Part model, mm, in its own coordinate system. Face numbers are marked on the shaded views. Round coordinates to 2 decimals unless told otherwise and drop trailing zeros. Write each loop counter-clockwise with the first axis right and the second up, starting at its lowest first coordinate (ties: lowest second). Pieces come first, ordered by that corner, then holes. Notation, with made-up numbers: M 2.25,65.5 L 56.25,65.5 A25 ccw 56.25,88.5 Z; hole C 7.5,56 d8. An arc over 180 degrees is marked long. Use one line per item in the form item = value. Start each with the question number.
Item 1: Probe L1, parallel to X at y = 4, z = -9.5; L2, parallel to Y at x = 26, z = 26; L3, parallel to Z at x = 29, y = 6. List the from-to ranges inside material, lowest first.
Item 2: Flat gauge pins, fed straight in: pin 1 Ø6 at (x, z) = (-36, 11) entering from +Y; pin 2 Ø8 at (x, z) = (4, -23.5) entering from +Y; pin 3 Ø3 at (x, y) = (20.5, 12) entering from +Z. Where does each tip first touch, or does it go through?
Item 3: Cut at A-A, the plane y = 40. Give the cut face in (x, z).
Item 4: Cut at B-B, the plane z = -63. Give the cut face in (x, y), then the cut area to 3 significant figures.
Item 5: Mould opens along X. For the marked faces 1, 2, 3 and 4 say: +X half, -X half, draft (parallel to the pull), parting line (faces both ways), or undercut.
from build123d import *

# Parameters (mm, degrees)
SKETCH1_W           = 84
SKETCH1_H           = 155
BOSS_EXTRUDE1_DEPTH = 3
SKETCH2_W           = 3
SKETCH2_H           = 3
CUT_EXTRUDE1_DEPTH  = 3
SKETCH3_W           = 5
SKETCH3_H           = 8
BOSS_EXTRUDE2_DEPTH = 155
SKETCH4_W           = 5
SKETCH4_H           = 8
BOSS_EXTRUDE3_DEPTH = 155
SKETCH5_W           = 5
SKETCH5_H           = 58
BOSS_EXTRUDE4_DEPTH = 84
BOSS_EXTRUDE5_DEPTH = 5
BOSS_EXTRUDE6_DEPTH = 5
SKETCH8_W           = 84
SKETCH8_H           = 8
BOSS_EXTRUDE8_DEPTH = 5
SKETCH10_W          = 10
SKETCH10_H          = 7.49718506
CUT_EXTRUDE2_DEPTH  = 5
SKETCH11_W          = 10
SKETCH11_H          = 10.666578164
CUT_EXTRUDE3_DEPTH  = 5
SKETCH12_W          = 2.991300293
SKETCH12_H          = 5
CUT_EXTRUDE4_DEPTH  = 1.5
CUT_EXTRUDE5_DEPTH  = 1.5


with BuildPart() as part:
    # Sketch1 → Boss-Extrude1 (new body)
    with BuildSketch(Plane(origin=(0, 0, 0), x_dir=(1, 0, 0), z_dir=(0, 1, 0))):
        Rectangle(SKETCH1_W, SKETCH1_H)
    extrude(amount=BOSS_EXTRUDE1_DEPTH)

    # Sketch2 → Cut-Extrude1 (cut)
    with BuildSketch(Plane(origin=(0, 3, 0), x_dir=(1, 0, 0), z_dir=(0, 1, 0))):
        with Locations((35.5, -71)):
            Rectangle(SKETCH2_W, SKETCH2_H)
        with Locations((-35.5, -71)):
            Rectangle(SKETCH2_W, SKETCH2_H)
    extrude(amount=-CUT_EXTRUDE1_DEPTH, mode=Mode.SUBTRACT)

    # Sketch3 → Boss-Extrude2 (add)
    with BuildSketch(Plane.XY.offset(77.5)):
        with Locations((39.5, 4)):
            Rectangle(SKETCH3_W, SKETCH3_H)
    extrude(amount=-BOSS_EXTRUDE2_DEPTH)

    # Sketch4 → Boss-Extrude3 (add)
    with BuildSketch(Plane.XY.offset(77.5)):
        with Locations((-39.5, 4)):
            Rectangle(SKETCH4_W, SKETCH4_H)
    extrude(amount=-BOSS_EXTRUDE3_DEPTH)

    # Sketch5 → Boss-Extrude4 (add)
    with BuildSketch(Plane.ZY.offset(42)):
        with Locations((-75, 29)):
            Rectangle(SKETCH5_W, SKETCH5_H)
    extrude(amount=-BOSS_EXTRUDE4_DEPTH)

    # Sketch6 → Boss-Extrude5 (add)
    with BuildSketch(Plane.ZY.offset(42)):
        Polygon((-72.5, 58), (-22.5, 8), (-74.300026141, 4.41684906), (-74.300026141, 56.199973859), align=None)
    extrude(amount=-BOSS_EXTRUDE5_DEPTH)

    # Sketch7 → Boss-Extrude6 (add)
    with BuildSketch(Plane(origin=(42, 0, 0), x_dir=(0, 0, -1), z_dir=(1, 0, 0))):
        Polygon((72.5, 58), (19.108860597, 4.608860597), (75.247556584, 4.608860597), (75.247556584, 53.916409465), align=None)
    extrude(amount=-BOSS_EXTRUDE6_DEPTH)

    # Sketch8 → Boss-Extrude8 (add)
    with BuildSketch(Plane.XY.offset(77.5)):
        with Locations((0, 4)):
            Rectangle(SKETCH8_W, SKETCH8_H)
    extrude(amount=-BOSS_EXTRUDE8_DEPTH)

    # Sketch10 → Cut-Extrude2 (cut)
    with BuildSketch(Plane.XY.offset(77.5)):
        with Locations((-17, 6.74859253)):
            Rectangle(SKETCH10_W, SKETCH10_H)
    extrude(amount=-CUT_EXTRUDE2_DEPTH, mode=Mode.SUBTRACT)

    # Sketch11 → Cut-Extrude3 (cut)
    with BuildSketch(Plane.XY.offset(77.5)):
        with Locations((17, 8.333289082)):
            Rectangle(SKETCH11_W, SKETCH11_H)
    extrude(amount=-CUT_EXTRUDE3_DEPTH, mode=Mode.SUBTRACT)

    # Sketch12 → Cut-Extrude4 (cut)
    with BuildSketch(Plane(origin=(0, 0, 0), x_dir=(-1, 0, 0), z_dir=(0, -1, 0))):
        with Locations((35.504349854, -75)):
            Rectangle(SKETCH12_W, SKETCH12_H)
    extrude(amount=-CUT_EXTRUDE4_DEPTH, mode=Mode.SUBTRACT)

    # Sketch13 → Cut-Extrude5 (cut)
    with BuildSketch(Plane(origin=(0, 0, 0), x_dir=(-1, 0, 0), z_dir=(0, -1, 0))):
        Polygon((-34, -72.5), (-34, -80.193887821), (-37, -80.075389367), (-37, -72.5), align=None)
    extrude(amount=-CUT_EXTRUDE5_DEPTH, mode=Mode.SUBTRACT)


solid = part.part
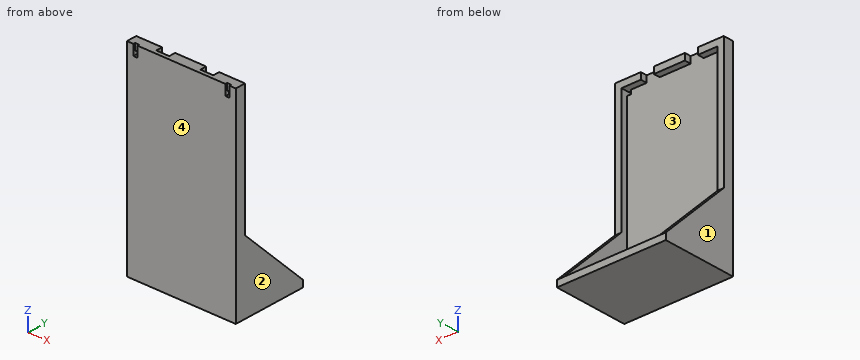
Model answer:
q1.L1 = -42 to -37, 37 to 42
q1.L2 = 0 to 3
q1.L3 = -77.5 to -72.5, 72.5 to 77.5
q2.pin_1 = 8
q2.pin_2 = 3
q2.pin_3 = -72.5
q3.outline = M -42,-77.5 L 42,-77.5 L 42,-54.5 L 37,-54.5 L 37,-72.5 L -37,-72.5 L -37,-54.5 L -42,-54.5 Z
q4.outline = M -42,0 L 42,0 L 42,48.5 L 37,48.5 L 37,3 L -37,3 L -37,48.5 L -42,48.5 Z
q4.area = 707 mm²
q5.face_1 = -X half
q5.face_2 = +X half
q5.face_3 = undercut
q5.face_4 = draft
